Could you check a few things on this model? Use its own coordinates, in mm. A direction names the side the tool comes from. Round coordinates to 2 decimals unless told otherwise and drop trailing zeros. Write each loop counter-clockwise with the first axis right and the second up, starting at its lowest first coordinate (ties: lowest second). Pieces come first, ordered by that corner, then holes. Notation, with made-up numbers: (85.5, 20.5) - (105.5, 20.5) arc R23 cw to (105.5, 55.5) - close; hole circle Ø2 at (41, 45). An arc over 180 degrees is marked (long way). Write each question's results on one line, items separated by ' | '. Start each with the question number.
(1) On a 3-axis mill with a long thin cutter (end or side, diameter ignored), from which of +Z, -Z, +X, -X, +Y, -Y can I reach the whole of each face in a straight line? I mean faces 4 (the flat face through (15, 0, 4)), 5 (the cylindrical face through (13.404, -1.998, 3.588)), 6 (the cylindrical face through (-13.404, -1.998, 3.588)). Say none if no direction works.
(2) Imagine slicing it at A-A on x = 0. Write out the boundary of the cut face in (y, z).
(3) Please list where these lines run through material, in increasing order: line 1 (X direction, y = 0, z = 3.8); line 2 (Y direction, x = 0, z = 3.3); line 3 (Y direction, x = 3.25, z = 2). Write a range as [from, to].
(4) Thinking about a two-plate mould opening in Y: for faces 1 (the cylindrical face through (11.923, 3.755, 3.458)), 2 (the cylindrical face through (-2.38, -10.74, 3.46)), 3 (the flat face through (6, -10, 0)), which applies, +Y half, -Y half, draft (parallel to the pull), parting line (faces both ways), or undercut?
(5) For P1, Ø4, axis at x = 5, z = 2, coming from the +Y side; P2, Ø1.5, axis at x = -2, z = 1.5, coming from the +Y side; P3, Ø1, axis at y = 7, z = 2, coming from the -X side; P4, Ø13, axis at x = 0, y = 0, coming from the +Z side, each with a flat end and sliding along its axis, tell me the tip position at first contact or that it passes through.
(6) Imagine slicing it at B-B on y = 0. Write out the boundary of the cut face in (x, z), then the cut area to 3 significant figures.
(7) Imagine slicing it at C-C on z = 3.5. Write out the boundary of the cut face in (x, y).
(8) Imagine slicing it at D-D on x = 13. Write out the boundary of the cut face in (y, z).
```python
from build123d import *

# Parameters (mm, degrees)
F0_R     = 12.5
F0_R_2   = 11
F1_DEPTH = 7
F2_SIZE  = 0.5
F4_R     = 2
F5_DEPTH = 4
F7_SIZE  = 0.5


with BuildPart() as f1:
    # F0 (on Top) → F1 (new body)
    with BuildSketch(Plane.XY):
        Circle(F0_R)
        Circle(F0_R_2, mode=Mode.SUBTRACT)
    extrude(amount=F1_DEPTH)

    # F2
    f2_edges = [f1.edges().sort_by_distance(p)[0] for p in [
        (-11, 0, 7),
        (-12.5, 0, 7),
        (-12.5, 0, 0),
        (-11, 0, 0),
    ]]
    chamfer(f2_edges, length=F2_SIZE)

    # F4 (on offset) → F5 (join)
    with BuildSketch(Plane.YZ.offset(11)):
        with Locations((0, 3.5)):
            Circle(F4_R)
    extrude(amount=F5_DEPTH)

    # F6: F1 across plane


with BuildPart() as f1_1:
    add(f1.part)
    add(f1.part.mirror(Plane.YZ))

    # F7
    f7_edges = [f1_1.edges().sort_by_distance(p)[0] for p in [
        (15, -2, 3.5),
        (-15, -2, 3.5),
    ]]
    chamfer(f7_edges, length=F7_SIZE)


solid = f1_1.part
```
Response:
1) face 4: +Z, -Z, +X, +Y, -Y | face 5: +X | face 6: -X
2) outline: (-12.5, 0.5) - (-12, 0) - (-11.5, 0) - (-11, 0.5) - (-11, 6.5) - (-11.5, 7) - (-12, 7) - (-12.5, 6.5) - close; (11, 0.5) - (11.5, 0) - (12, 0) - (12.5, 0.5) - (12.5, 6.5) - (12, 7) - (11.5, 7) - (11, 6.5) - close
3) line 1: [-15, -11], [11, 15] | line 2: [-12.5, -11], [11, 12.5] | line 3: [-12.07, -10.51], [10.51, 12.07]
4) face 1: parting line | face 2: undercut | face 3: draft
5) P1: y = 12.13 | P2: y = 12.44 | P3: x = -10.68 | P4: through
6) outline: (-15, 2) - (-14.5, 1.5) - (-12.5, 1.5) - (-12.5, 0.5) - (-12, 0) - (-11.5, 0) - (-11, 0.5) - (-11, 6.5) - (-11.5, 7) - (-12, 7) - (-12.5, 6.5) - (-12.5, 5.5) - (-14.5, 5.5) - (-15, 5) - close; (11, 0.5) - (11.5, 0) - (12, 0) - (12.5, 0.5) - (12.5, 1.5) - (14.5, 1.5) - (15, 2) - (15, 5) - (14.5, 5.5) - (12.5, 5.5) - (12.5, 6.5) - (12, 7) - (11.5, 7) - (11, 6.5) - close | area: 39.5 mm²
7) outline: (-15, -1.5) - (-14.5, -2) - (-12.34, -2) arc R12.5 ccw to (12.34, -2) - (14.5, -2) - (15, -1.5) - (15, 1.5) - (14.5, 2) - (12.34, 2) arc R12.5 ccw to (-12.34, 2) - (-14.5, 2) - (-15, 1.5) - close; hole circle Ø22 at (0, 0)
8) outline: circle Ø4 at (0, 3.5)
